Can you work these out from the model? Positions are in its coordinate system, mm. A direction names the side the tool comes from. Give positions to 0.01 mm unless a question says otherwise; leave off trailing zeros. Order: outer loops, then holes, each group sorted by start corner. A loop starts at its lowest first (then second) coordinate and runs counter-clockwise, first axis right, second up. Notation, with made-up numbers: (-32, 57.5) - (17, 57.5) arc R32 cw to (17, 92.5) - close; hole circle Ø9 at (53.25, -39.5). An arc over 180 degrees is marked (long way). Return JSON: item names as keys, results as strings.
Autodesk Inventor part; units mm, degrees
ref_plane "YZ Plane" through (0, 0, 0) normal (1, 0, 0) x (0, 1, 0)
ref_plane "XZ Plane" through (0, 0, 0) normal (0, 1, 0) x (-1, 0, 0)
ref_plane "XY Plane" through (0, 0, 0) normal (0, 0, 1) x (1, 0, 0)
sketch "Sketch1" plane through (0, 0, 0) normal (0, 0, 1) x (1, 0, 0)
  circle A0 centre (0, 0) radius 2.125
  circle A1 centre (0, 0) radius 6
  line L0 (0, 0) -> (0, 6) construction
  line L1 (3.75, 0) -> (3.75, 6)
  line L2 (-3.75, 6) -> (-3.75, 0)
  arc A2 (-3.75, 0) -> (3.75, 0) centre (0, 0) ccw
  arc A3 (3.75, 6) -> (-3.75, 6) centre (0, 6) ccw construction
  line L3 (0, 0) -> (-6, 0) construction
  line L4 (0, 3.75) -> (-6, 3.75)
  line L5 (-6, -3.75) -> (0, -3.75)
  arc A4 (0, -3.75) -> (0, 3.75) centre (0, 0) ccw
  arc A5 (-6, 3.75) -> (-6, -3.75) centre (-6, 0) ccw construction
  circle A6 centre (0, 12.35) radius 6.35 construction
  circle A7 centre (0, 10.1) radius 6.35 construction
  arc A8 (3.75, 4.6837) -> (-4.6837, -3.75) centre (2.5103, -2.5103) ccw
  point P0 (0, 3)
  point P1 (-3, 0)
  point P2 (0, -3.75)
  point P3 (-4.6837, -3.75)
  point P4 (-3.75, 4.6837)
  point P5 (-3.75, 3.75)
  point P6 (-4.6837, 3.75)
  dimension "d0" = 4.25
  dimension "d3" = 12
  dimension "d4" = 7.5
  dimension "d5" = 7.5
  dimension "d6" = 90
  dimension "d7" = 12.7
  dimension "d8" = 12.7
extrude "Extrusion1" add sketch "Sketch1" along normal blind 3.175
extrude "Extrusion2" add sketch "Sketch1" along normal blind 7.9375 contours A1 L5 A2 L1
fillet "Fillet1" radius 1 2 edges at (3.75, 4.6837, 5.5563) (-4.6837, -3.75, 5.5563)
equation "\"d4\" = d5"
properties part number "Cam - Shell" material "Nylon 6/6"
1. On a 3-axis mill with a long thin cutter (end or side, diameter ignored), from which of +Z, -Z, +X, -X, +Y, -Y can I reach the whole of each face in a straight line? I mean faces 1 (the face through (3.226, -5.059, 3.031)), 2 (the face through (4.61, 2.55, 5.59)), 3 (the face through (3.75, 1, 6)). Say none if no direction works.
Checks:
{"face 1": "+Z, -Z", "face 2": "+Z, +Y", "face 3": "+Z, -X, +Y"}
2. Suppose I cut it at D-D (y = -2.5). List the corners of the cut face in (x, z) for me (1 decimal).
Checks:
{"outline": "(-5.5, 0) - (5.5, 0) - (5.5, 7.9) - (2.8, 7.9) - (2.8, 3.2) - (-5.5, 3.2) - close"}
3. Suppose I cut it at B-B (z = 2.25). List the corners of the cut face in (x, y) for me (3 decimals).
Checks:
{"outline": "circle Ø12 at (0, 0); hole circle Ø4.25 at (0, 0)"}
4. Suppose I cut it at A-A (y = -1). List the corners of the cut face in (x, z) for me (1 decimal).
Checks:
{"outline": "(-5.9, 0) - (-1.9, 0) - (-1.9, 3.2) - (-5.9, 3.2) - close; (1.9, 0) - (5.9, 0) - (5.9, 7.9) - (3.6, 7.9) - (3.6, 3.2) - (1.9, 3.2) - close"}
5. Thinking about a two-plate mould opening in Y: for faces 4 (the face through (-2.545, -4.572, 5.59)), 5 (the face through (3, 0, 0)), 6 (the face through (1.142, -1.792, 1.565)), which applies, +Y half, -Y half, draft (parallel to the pull), parting line (faces both ways), or undercut?
Checks:
{"face 4": "parting line", "face 5": "draft", "face 6": "undercut"}
6. For pin 1 Ø1.7 at (y, z) = (0.5, 4.5) entering from -X; pin 2 Ø2 at (x, z) = (2.5, 4) entering from -Y; pin 3 Ø1 at (x, z) = (1.5, 2) entering from -Y, each with a flat end and sliding along its axis, tell me the tip position at first contact or that it passes through.
Checks:
{"pin 1": "x = 3.73", "pin 2": "y = -5.81", "pin 3": "y = -5.92"}
7. If I drill on L1, parallel to Y at x = 0, z = 1.9 (3 decimals); L2, parallel to Y at x = -1, z = 1 (3 decimals); L3, parallel to Z at x = -5.25, y = 2.5 (3 decimals), over which ranges is the centre line in solid material (lowest first)? Write a range as [from, to].
Checks:
{"L1": "[-6, -2.125], [2.125, 6]", "L2": "[-5.916, -1.875], [1.875, 5.916]", "L3": "[0, 3.175]"}
